The model under review builds one solid part; all positions refer to its coordinate system, in mm. Face numbers are marked on the shaded views. A direction names the side the tool comes from. Round coordinates to 2 decimals unless told otherwise and drop trailing zeros. Order: outer loops, then holes, each group sorted by start corner. A loop starts at its lowest first (then second) coordinate and runs counter-clockwise, first axis right, second up. Notation, with made-up numbers: (-1.75, 2) -> (22.25, 2) arc R9 cw to (22.25, 6) -> close; hole circle Ø9 at (60, -16). An arc over 180 degrees is marked (long way). Return JSON: item names as keys, results as strings. Group by question number.
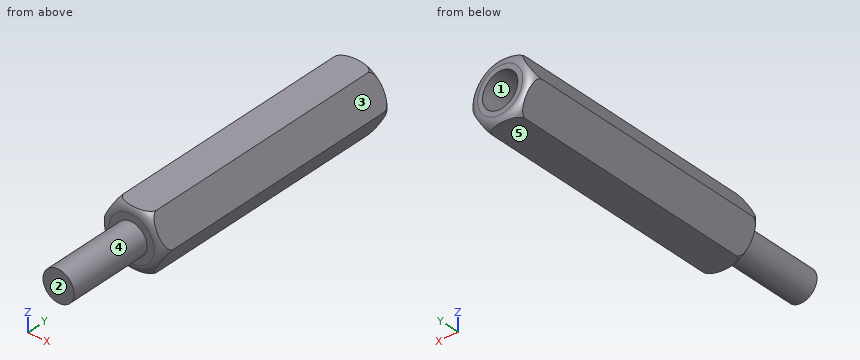
from build123d import *

# Parameters (mm, degrees)
BOSS_EXTRUDE1_DEPTH      = 25
M3_CLEARANCE_HOLE1_D     = 3.4
M3_CLEARANCE_HOLE1_DEPTH = 12
M3_CLEARANCE_HOLE1_TIP   = 1.021463052
SKETCH5_R                = 1.5
BOSS_EXTRUDE2_DEPTH      = 8


with BuildPart() as part:
    # Sketch1 → Boss-Extrude1 (new body)
    with BuildSketch(Plane(origin=(0, 0, 0), x_dir=(1, 0, 0), z_dir=(0, 1, 0))):
        Polygon((3.175426481, 0), (1.58771324, 2.75), (-1.58771324, 2.75), (-3.175426481, 0), (-1.58771324, -2.75), (1.58771324, -2.75), align=None)
    extrude(amount=BOSS_EXTRUDE1_DEPTH)

    # M3 Clearance Hole1
    with Locations(Plane(origin=(0, 25, 0), x_dir=(-1, 0, 0), z_dir=(0, 1, 0))):
        with Locations((0, 0)):
            Hole(M3_CLEARANCE_HOLE1_D / 2, depth=M3_CLEARANCE_HOLE1_DEPTH)
            with Locations((0, 0, -(M3_CLEARANCE_HOLE1_DEPTH + M3_CLEARANCE_HOLE1_TIP / 2))):  # 118° drill point
                Cone(0, M3_CLEARANCE_HOLE1_D / 2, M3_CLEARANCE_HOLE1_TIP, mode=Mode.SUBTRACT)

    # Sketch4 → Cut-Revolve1 (revolve, cut)
    with BuildSketch(Plane.XY):
        with BuildLine():
            Line((-2.175426481, 25), (-3.175426481, 25))
            Line((-3.175426481, 25), (-3.175426481, 24))
            ThreePointArc((-3.175426481, 24), (-2.882533262, 24.707106781), (-2.175426481, 25))
        make_face()
        with BuildLine():
            Line((-3.175426481, 1), (-3.175426481, 0))
            Line((-3.175426481, 0), (-2.175426481, 0))
            ThreePointArc((-2.175426481, 0), (-2.882533262, 0.292893219), (-3.175426481, 1))
        make_face()
    revolve(axis=Axis((0, 25, 0), (0, -1, 0)), mode=Mode.SUBTRACT)

    # Sketch5 → Boss-Extrude2 (add)
    with BuildSketch(Plane.XZ):
        Circle(SKETCH5_R)
    extrude(amount=BOSS_EXTRUDE2_DEPTH)


solid = part.part
Item 1: For the marked faces 4 and 5, list the 3-axis set-ups (+Z, -Z, +X, -X, +Y, -Y) from which the entire face can be reached by the end or side of a thin tool; tool diameter is ignored.
Item 2: Wall thickness on line 1 along Z through (x, y) = (0, 16.75); line 2 along Y through (x, z) = (2.75, -0.2); line 3 along Z through (x, y) = (-1.5, 13.5): over which ranges is each line inside the solid? List them lowest first.
Item 3: The part is to be moulded in two halves that separate along Z. For the marked faces 1, 2 and 3, say which applies: +Z half, -Z half, draft (parallel to the pull), parting line (faces both ways), or undercut.
Item 4: Insertion check: pin 1 Ø1.5 at (y, z) = (-3, 2) entering from -X; pin 2 Ø1 at (y, z) = (13, -1.5) entering from -X. Each pin has a flat end and moves straight along its axis. Give the tip position at first contact, or say it passes through.
Item 5: Consider section B-B on y = -5.5. State the section outline as (x, z) points.
Item 6: Consider section A-A on y = 15.5. State the section outline as (x, z) points.
Values:
{
 "1": {"face 4": "-Y", "face 5": "-Z, +X, -X, +Y, -Y"},
 "2": {"line 1": "-2.75 to -1.7, 1.7 to 2.75", "line 2": "0.19 to 24.81", "line 3": "-2.75 to -0.8, 0.8 to 2.75"},
 "3": {"face 1": "undercut", "face 2": "draft", "face 3": "+Z half"},
 "4": {"pin 1": "x = -0.83", "pin 2": "x = -2.6"},
 "5": {"outline": "circle Ø3 at (0, 0)"},
 "6": {"outline": "(-3.18, 0) -> (-1.59, -2.75) -> (1.59, -2.75) -> (3.18, 0) -> (1.59, 2.75) -> (-1.59, 2.75) -> close; hole circle Ø3.4 at (0, 0)"}
}
